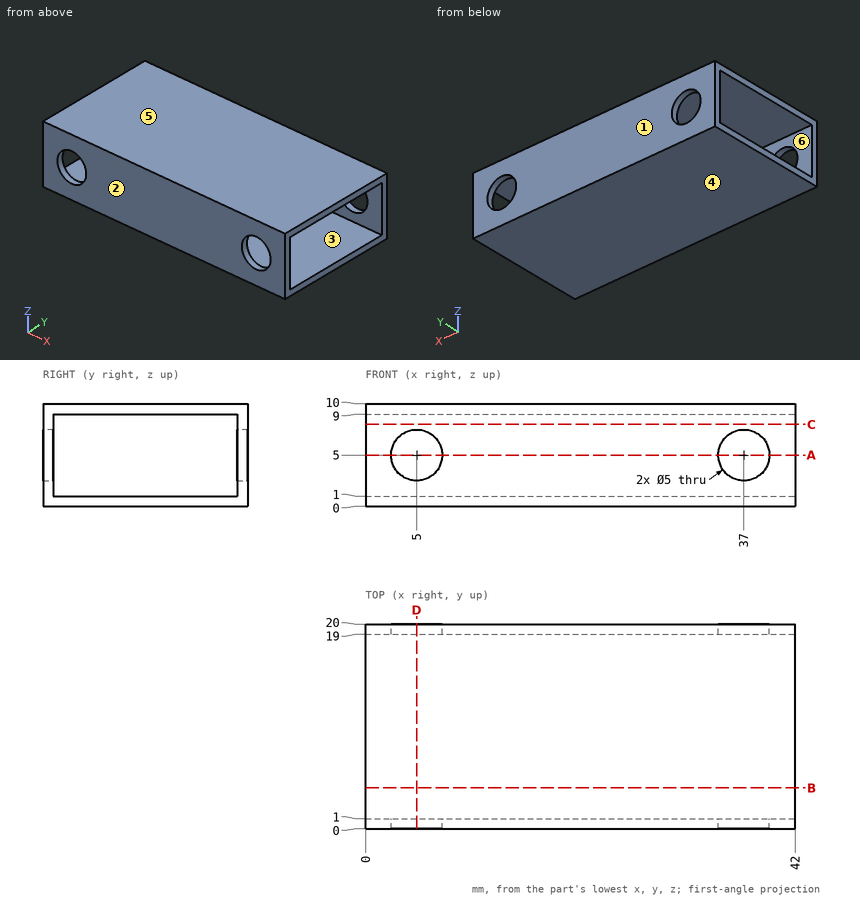
Verification items for this drawing (mm, ordinates from the low corner). A direction names the side the tool comes from. Coordinates: 2 decimals unless noted, no trailing zeros. Write each loop counter-clockwise with the first axis right and the second up, starting at its lowest first coordinate (ties: lowest second). Pieces come first, ordered by that corner, then holes. Notation, with made-up numbers: M -11,27 L 38,27 A30 ccw 38,57 Z; hole C 81,-27 d1. An arc over 180 degrees is marked long. One line per item, written item: value. Start each with the question number.
(1) Sectioned sample at D-D, the plane x = 5. Enter the section's corners in (y, z).
(2) Depth check by flat-ended pin: pin 1 (4 mm diameter, centred on x = 5, z = 5, fed in from +Y); pin 2 (5 mm diameter, centred on y = 3, z = 4, fed in from +X). Enter the tip coordinate at first touch or a pass-through.
(3) Scan lines: line 1 along X through (y, z) = (19.55, 5); line 2 along Y through (x, z) = (26.5, 1.5); line 3 along Z through (x, y) = (14, 8.25). Record each from-to range of solid material in increasing order. Write a range as [from, to].
(4) Sectioned sample at B-B, the plane y = 4. Enter the section's corners in (x, z), and give its area (3 significant figures).
(5) Tool access check on the marked faces 5 and 6. Record the directions out of +Z, -Z, +X, -X, +Y, -Y that give a thin tool (end or side, any length) a straight path to the whole face; none if there is none.
(6) Release check for a two-part mould opening along Y. For the marked faces 1, 2, 3 and 4 record: released by +Y, released by -Y, zero draft, split by the parting line, or undercut.
(7) Sectioned sample at A-A, the plane z = 5. Enter the section's corners in (x, y).
(8) Sectioned sample at C-C, the plane z = 8. Enter the section's corners in (x, y).
Filled sheet:
1. outline: M 0,0 L 20,0 L 20,2.5 L 19,2.5 L 19,1 L 1,1 L 1,2.5 L 0,2.5 Z; M 0,7.5 L 1,7.5 L 1,9 L 19,9 L 19,7.5 L 20,7.5 L 20,10 L 0,10 Z
2. pin 1: through
2. pin 2: x = 42
3. line 1: [0, 2.5], [7.5, 34.5], [39.5, 42]
3. line 2: [0, 1], [19, 20]
3. line 3: [0, 1], [9, 10]
4. outline: M 0,0 L 42,0 L 42,1 L 0,1 Z; M 0,9 L 42,9 L 42,10 L 0,10 Z
4. area: 84.0 mm²
5. face 5: +Z, +X, -X, +Y, -Y
5. face 6: +X, -X
6. face 1: released by +Y
6. face 2: released by -Y
6. face 3: undercut
6. face 4: zero draft
7. outline: M 0,0 L 2.5,0 L 2.5,1 L 0,1 Z; M 0,19 L 2.5,19 L 2.5,20 L 0,20 Z; M 7.5,0 L 34.5,0 L 34.5,1 L 7.5,1 Z; M 7.5,19 L 34.5,19 L 34.5,20 L 7.5,20 Z; M 39.5,0 L 42,0 L 42,1 L 39.5,1 Z; M 39.5,19 L 42,19 L 42,20 L 39.5,20 Z
8. outline: M 0,0 L 42,0 L 42,1 L 0,1 Z; M 0,19 L 42,19 L 42,20 L 0,20 Z
